```python
from build123d import *

# Parameters (mm, degrees)
SWEEP1_PROFILE_R = 5.588


with BuildPart() as part:
    # Sweep1: sweep along a path in Sketch1
    with BuildLine(Plane.XY) as sweep1_path:
        Line((0, 0), (23.622, 0))
        ThreePointArc((23.622, 0), (29.714292142, -1.581578377), (34.267947791, -5.92687859))
        Line((34.267947791, -5.92687859), (48.006, -28.09416816))
        ThreePointArc((48.006, -28.09416816), (53.546892782, -33.381533837), (60.96, -35.306))
        ThreePointArc((60.96, -35.306), (88.259978608, -23.997978608), (99.568, 3.302))
        ThreePointArc((99.568, 3.302), (95.029912468, 14.257912468), (84.074, 18.796))
        Line((84.074, 18.796), (-14.986, 18.796))
    # Sweep1 profile (on start of the path) → Sweep1 (sweep)
    with BuildSketch(Plane.YZ):
        Circle(SWEEP1_PROFILE_R)
    sweep(path=sweep1_path.line)


solid = part.part
```
Check sheet for the modelled part. Datum: model origin and axes. Units: mm. A direction names the side the tool comes from. Round coordinates to 2 decimals unless told otherwise and drop trailing zeros. Loops run counter-clockwise (first coordinate to the right, second up) from the corner with the lowest first, then second, coordinate; pieces in that order, holes last. Notation, with made-up numbers: (84.5, 55.5) -> (141.5, 55.5) arc R15 ccw to (141.5, 78.5) -> close; hole circle Ø8 at (32, -15). An arc over 180 degrees is marked (long way). Write item = value, one per line. Start each with the question number.
1) Thickness scan on probe 1 along Y at (x, z) = (85, 2.25); probe 2 along Y at (x, z) = (38, 0.5); probe 3 along X at (y, z) = (-7.5, 2.75). Record the ranges inside material, lowest first.
2) Sectioned sample at A-A, the plane z = 3.25. Record the cut outline in (x, y).
3) Gauge pin test, flat ends, axial feed: pin 1 Ø5.5 at (y, z) = (0.5, 0) entering from -X; pin 2 Ø6 at (x, z) = (12.5, 0.5) entering from -Y; pin 3 Ø1 at (x, y) = (20.5, 17) entering from +Z. Record the tip position at first contact, or that the pin passes through.
4) Set-up check for faces 1 (the flat face through (-14.986, 19, 0)), 2 (the cylindrical face through (11.976, -4.434, -3.4)): record each of +Z, -Z, +X, -X, +Y, -Y from which the full face is reachable in a straight line by a thin tool's end or side.
5) Release check for a two-part mould opening along Y. For faces 3 (the flat face through (0, 0, 0)), 4 (the cylindrical face through (33.85, 24.38, 0.25)) record: released by +Y, released by -Y, zero draft, split by the parting line, or undercut.
6) Sectioned sample at B-B, the plane z = -1.75. Record the cut outline in (x, y).
Results are:
q1.probe_1 = -33.22 to -20.02, 13.64 to 23.89
q1.probe_2 = -22.51 to -1.55, 13.23 to 24.36
q1.probe_3 = 29.4 to 40.97, 92.93 to 103.07
q2.outline = (-14.99, 14.25) -> (84.07, 14.25) arc R10.95 cw to (95.02, 3.3) arc R34.06 cw to (60.96, -30.76) arc R10.69 cw to (51.87, -25.7) -> (38.13, -3.53) arc R17.07 ccw to (23.62, 4.55) -> (0, 4.55) -> (0, -4.55) -> (23.62, -4.55) arc R7.98 cw to (30.4, -8.32) -> (44.14, -30.49) arc R19.79 ccw to (60.96, -39.85) arc R43.15 ccw to (104.11, 3.3) arc R20.04 ccw to (84.07, 23.34) -> (-14.99, 23.34) -> close
q3.pin_1 = 0
q3.pin_2 = -5.59
q3.pin_3 = 5.44
q4.face_1 = +Z, -Z, -X, +Y, -Y
q4.face_2 = -X
q5.face_3 = zero draft
q5.face_4 = undercut
q6.outline = (-14.99, 13.49) -> (84.07, 13.49) arc R10.19 cw to (94.26, 3.3) arc R33.3 cw to (60.96, -30) arc R9.93 cw to (52.52, -25.3) -> (38.78, -3.13) arc R17.83 ccw to (23.62, 5.31) -> (0, 5.31) -> (0, -5.31) -> (23.62, -5.31) arc R7.22 cw to (29.76, -8.72) -> (43.5, -30.89) arc R20.55 ccw to (60.96, -40.61) arc R43.91 ccw to (104.87, 3.3) arc R20.8 ccw to (84.07, 24.1) -> (-14.99, 24.1) -> close
